Can you work these out from the model? Positions are in its coordinate system, mm. Face numbers are marked on the shaded views. A direction names the side the tool comes from. Round coordinates to 2 decimals unless told otherwise and drop trailing zeros. Order: outer loops, then holes, each group sorted by start corner. A loop starts at its lowest first (then second) coordinate and runs counter-clockwise, first axis right, second up.
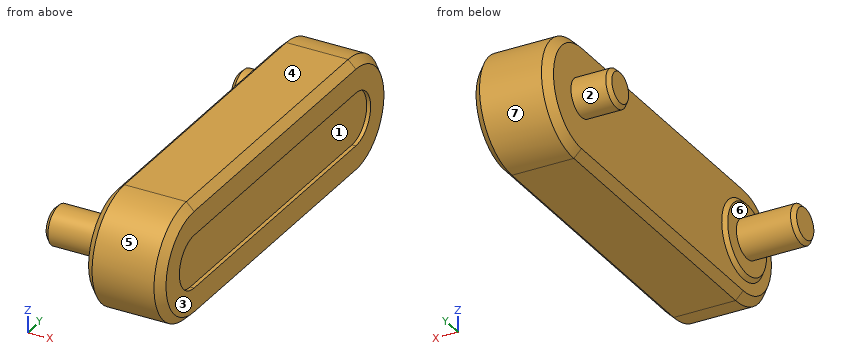
from build123d import *

# Parameters (mm, degrees)
SKETCH_1_R          = 4.9
EXTRUDE_1_DEPTH     = 10
EXTRUDE_2_DEPTH     = 20
SKETCH_3_R          = 5
EXTRUDE_3_DEPTH     = 16
CHAMFER_1_SIZE      = 2
CUT_EXTRUDE_1_DEPTH = 1
SKETCH_5_R          = 10
EXTRUDE_4_DEPTH     = 1
CHAMFER_2_SIZE      = 1
CHAMFER_3_SIZE      = 1


with BuildPart() as part:
    # 草图1 → 凸台-拉伸1 (new body)
    with BuildSketch(Plane(origin=(0, 0, 0), x_dir=(0, 0, -1), z_dir=(1, 0, 0))):
        Circle(SKETCH_1_R)
    extrude(amount=EXTRUDE_1_DEPTH)

    # 草图2 → 凸台-拉伸2 (add)
    with BuildSketch(Plane(origin=(10, 0, 0), x_dir=(0, 0, -1), z_dir=(1, 0, 0))):
        with BuildLine():
            Line((15, 0), (15, -75))
            ThreePointArc((15, -75), (0, -90), (-15, -75))
            Line((-15, -75), (-15, 0))
            ThreePointArc((-15, 0), (0, 15), (15, 0))
        make_face()
    extrude(amount=EXTRUDE_2_DEPTH)

    # 草图3 → 凸台-拉伸3 (add)
    with BuildSketch(Plane.ZY.offset(-10)):
        with Locations(Location((0, -75, 0), (0, 0, 180))):
            Circle(SKETCH_3_R)
    extrude(amount=EXTRUDE_3_DEPTH)

    # 倒角1
    chamfer_1_edges = [part.edges().sort_by_distance(p)[0] for p in [
        (10, -37.5, 15),
        (10, -90, 0),
        (30, -37.5, -15),
        (10, 15, 0),
        (30, -37.5, 15),
        (30, -90, 0),
        (30, 15, 0),
        (10, -37.5, -15),
    ]]
    chamfer(chamfer_1_edges, length=CHAMFER_1_SIZE)

    # 草图4 → 切除-拉伸1 (cut)
    with BuildSketch(Plane(origin=(30, 0, 0), x_dir=(0, 0, -1), z_dir=(1, 0, 0))):
        with BuildLine():
            Line((6.835634275, 0), (6.835634275, -75))
            ThreePointArc((6.835634275, -75), (0, -81.835634275), (-6.835634275, -75))
            Line((-6.835634275, -75), (-6.835634275, 0))
            ThreePointArc((-6.835634275, 0), (0, 6.835634275), (6.835634275, 0))
        make_face()
    extrude(amount=-CUT_EXTRUDE_1_DEPTH, mode=Mode.SUBTRACT)

    # 草图5 → 凸台-拉伸4 (add)
    with BuildSketch(Plane.ZY.offset(-10)):
        with Locations(Location((0, -75, 0), (0, 0, 180))):
            Circle(SKETCH_5_R)
    extrude(amount=EXTRUDE_4_DEPTH)

    # 倒角2
    chamfer_2_edges = [part.edges().sort_by_distance(p)[0] for p in [
        (9, -75, 10),
    ]]
    chamfer(chamfer_2_edges, length=CHAMFER_2_SIZE - 0.0001)  # a hair under: the kernel refuses the full size

    # 倒角3
    chamfer_3_edges = [part.edges().sort_by_distance(p)[0] for p in [
        (-6, -75, 5),
        (0, 0, 4.9),
    ]]
    chamfer(chamfer_3_edges, length=CHAMFER_3_SIZE)


solid = part.part
(1) I want a section at C-C, the plane x = 25. List the corners of the cut face in (y, z) for me.
(2) On a 3-axis mill with a long thin cutter (end or side, diameter ignored), from which of +Z, -Z, +X, -X, +Y, -Y can I reach the whole of each face in a straight line? I mean the marked faces 1, 2 and 3. Say none if no direction works.
(3) I want a section at D-D, the plane x = 5. List the corners of the cut face in (y, z) for me.
(4) I want a section at B-B, the plane y = -50. List the corners of the cut face in (x, z) for me, plus the area to 3 significant figures.
(5) I'm going to push flat-ended pins straight in: pin 1 Ø15 at (y, z) = (-57, 0) entering from +X; pin 2 Ø12 at (x, z) = (2.5, 7.5) entering from +Y; pin 3 Ø6 at (y, z) = (2, 1.5) entering from -X; pin 4 Ø0.5 at (x, y) = (29.5, -40.5) entering from -Z. Where does each tip first touch, or does it pass through?
(6) If we mould it in two halves opening along Y, with no side actions, what happens to the marked faces 4, 5, 6 and 7? For each: pulls with the +Y half, pulls with the -Y half, needs draft (parallel to the pull), parting line crosses it, or undercut.
(7) Please list where these lines run through material, in increasing order: probe 1 along Y at (x, z) = (14.5, -12); probe 2 along X at (y, z) = (-78, 12.5); probe 3 along X at (y, z) = (-50, -3).
Ans:
1. outline: (-75, -15) - (0, -15) arc R15 ccw to (0, 15) - (-75, 15) arc R15 ccw to start
2. face 1: +X
2. face 2: -X
2. face 3: +Z, -Z, +X, +Y, -Y
3. outline: circle Ø10 at (-75, 0); circle Ø9.8 at (0, 0)
4. outline: (10, -13) - (12, -15) - (28, -15) - (30, -13) - (30, -6.84) - (29, -6.84) - (29, 6.84) - (30, 6.84) - (30, 13) - (28, 15) - (12, 15) - (10, 13) - close
4. area: 578 mm2
5. pin 1: stops at x = 30
5. pin 2: stops at y = 4.66
5. pin 3: stops at x = 0
5. pin 4: stops at z = -13.75
6. face 4: needs draft
6. face 5: pulls with the -Y half
6. face 6: undercut
6. face 7: pulls with the +Y half
7. probe 1: y = -84 to 9
7. probe 2: x = 10 to 30
7. probe 3: x = 10 to 29
